from build123d import *

# Parameters (mm, degrees)
SKETCH_1_W      = 32.5
SKETCH_1_H      = 16.8
SKETCH_1_R      = 4
EXTRUDE_1_DEPTH = 1.9
EXTRUDE_2_DEPTH = 3.75


with BuildPart() as part:
    # Эскиз1 → Бобышка-Вытянуть1 (new body)
    with BuildSketch(Plane.XY):
        Rectangle(SKETCH_1_W, SKETCH_1_H)
        Circle(SKETCH_1_R, mode=Mode.SUBTRACT)
    extrude(amount=EXTRUDE_1_DEPTH)

    # Эскиз3 → Бобышка-Вытянуть2 (add, symmetric)
    with BuildSketch(Plane(origin=(0, 0, 0), x_dir=(1, 0, 0), z_dir=(0, 1, 0))):
        with BuildLine():
            Line((-14.425, -8.710992724), (-7.45, -4.683974596))
            Line((-7.45, -4.683974596), (-6.5, -6.329422863))
            Line((-6.5, -6.329422863), (-13.475, -10.356440991))
            ThreePointArc((-13.475, -10.356440991), (-21.610888336, -6.9864457), (-16.25, 0))
            Line((-16.25, 0), (-16.25, -1.9))
            ThreePointArc((-16.25, -1.9), (-19.775629266, -6.494689515), (-14.425, -8.710992724))
        make_face()
    extrude_2 = extrude(amount=EXTRUDE_2_DEPTH, both=True)

    # Зеркальное отражение1: Бобышка-Вытянуть2 across plane
    add(extrude_2.mirror(Plane(origin=(0, 0, 0), x_dir=(0, 0, 1), z_dir=(1, 0, 0))))


solid = part.part
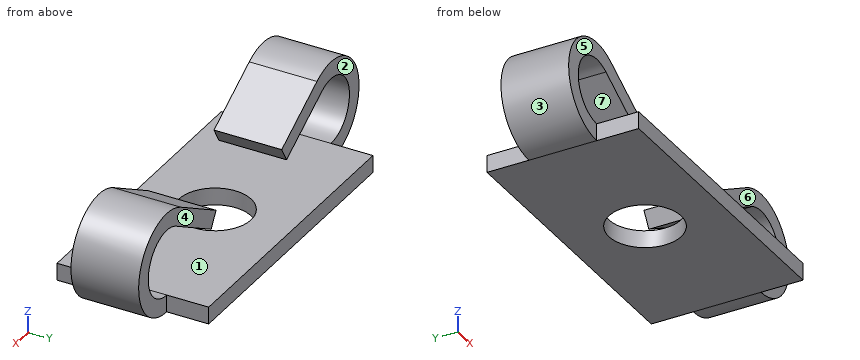
Here's how the part is built. I have some questions about the finished solid (model axes, mm). Face numbers are marked on the shaded views. A direction names the side the tool comes from. Round coordinates to 2 decimals unless told otherwise and drop trailing zeros. Order: outer loops, then holes, each group sorted by start corner. A loop starts at its lowest first (then second) coordinate and runs counter-clockwise, first axis right, second up. Notation, with made-up numbers: M 63.5,86.25 L 112.5,86.25 A24 cw 112.5,102.25 Z; hole C 81.25,35.5 d6. An arc over 180 degrees is marked long. Return JSON: item names as keys, results as strings. Group by question number.
1. If we section it at C-C on y = -6.75: List the corners of the cut face in (x, z) for me, then the cut area to 4 significant figures.
2. If we mould it in two halves opening along Z, with no side actions, what happens to the marked faces 1, 2 and 3? For each: pulls with the +Z half, pulls with the -Z half, needs draft (parallel to the pull), parting line crosses it, or undercut.
3. Please list where these lines run through material, in increasing order: probe 1 along Y at (x, z) = (0, 1); probe 2 along X at (y, z) = (-1.5, 5.55); probe 3 along X at (y, z) = (0.75, 8).
4. If we section it at A-A on x = 0: List the corners of the cut face in (y, z) for me, then the cut area to 3 significant figures.
5. If we section it at D-D on x = -12: List the corners of the cut face in (y, z) for me.
6. I'm going to push flat-ended pins straight in: pin 1 Ø3 at (x, z) = (-7, 3) entering from +Y; pin 2 Ø6 at (y, z) = (0.5, 9) entering from +X; pin 3 Ø1.5 at (y, z) = (-7, 1) entering from +X; pin 4 Ø1 at (y, z) = (6.5, 0.5) entering from -X. Where does each tip first touch, or does it pass through?
7. If we section it at B-B on z = 5.25: List the corners of the cut face in (x, y) for me.
8. On a 3-axis mill with a long thin cutter (end or side, diameter ignored), from which of +Z, -Z, +X, -X, +Y, -Y can I reach the whole of each face in a straight line? I mean the marked faces 4, 5, 6 and 7. Say none if no direction works.
Reply:
{
 "1": {"outline": "M -16.25,0 L 16.25,0 L 16.25,1.9 L -16.25,1.9 Z", "area": "61.75 mm^2"},
 "2": {"face 1": "undercut", "face 2": "needs draft", "face 3": "parting line crosses it"},
 "3": {"probe 1": "-8.4 to -4, 4 to 8.4", "probe 2": "-21.8 to -19.9, -8.95 to -6.95, 6.95 to 8.95, 19.9 to 21.8", "probe 3": "-21.23 to -18.96, -13.19 to -9.39, 9.39 to 13.19, 18.96 to 21.23"},
 "4": {"outline": "M -8.4,0 L -4,0 L -4,1.9 L -8.4,1.9 Z; M 4,0 L 8.4,0 L 8.4,1.9 L 4,1.9 Z", "area": "16.7 mm^2"},
 "5": {"outline": "M -8.4,0 L 8.4,0 L 8.4,1.9 L -8.4,1.9 Z; M -3.75,7.31 L 3.75,7.31 L 3.75,9.5 L -3.75,9.5 Z"},
 "6": {"pin 1": "y = 8.4", "pin 2": "x = 21.78", "pin 3": "x = 16.25", "pin 4": "x = -16.25"},
 "7": {"outline": "M -21.79,-3.75 L -19.89,-3.75 L -19.89,3.75 L -21.79,3.75 Z; M -8.43,-3.75 L -7.12,-3.75 L -7.12,3.75 L -8.43,3.75 Z; M 7.12,-3.75 L 8.43,-3.75 L 8.43,3.75 L 7.12,3.75 Z; M 19.89,-3.75 L 21.79,-3.75 L 21.79,3.75 L 19.89,3.75 Z"},
 "8": {"face 4": "+Z, +X, +Y", "face 5": "+Z, -X, -Y", "face 6": "+Z, +X, -Y", "face 7": "+Y, -Y"}
}
